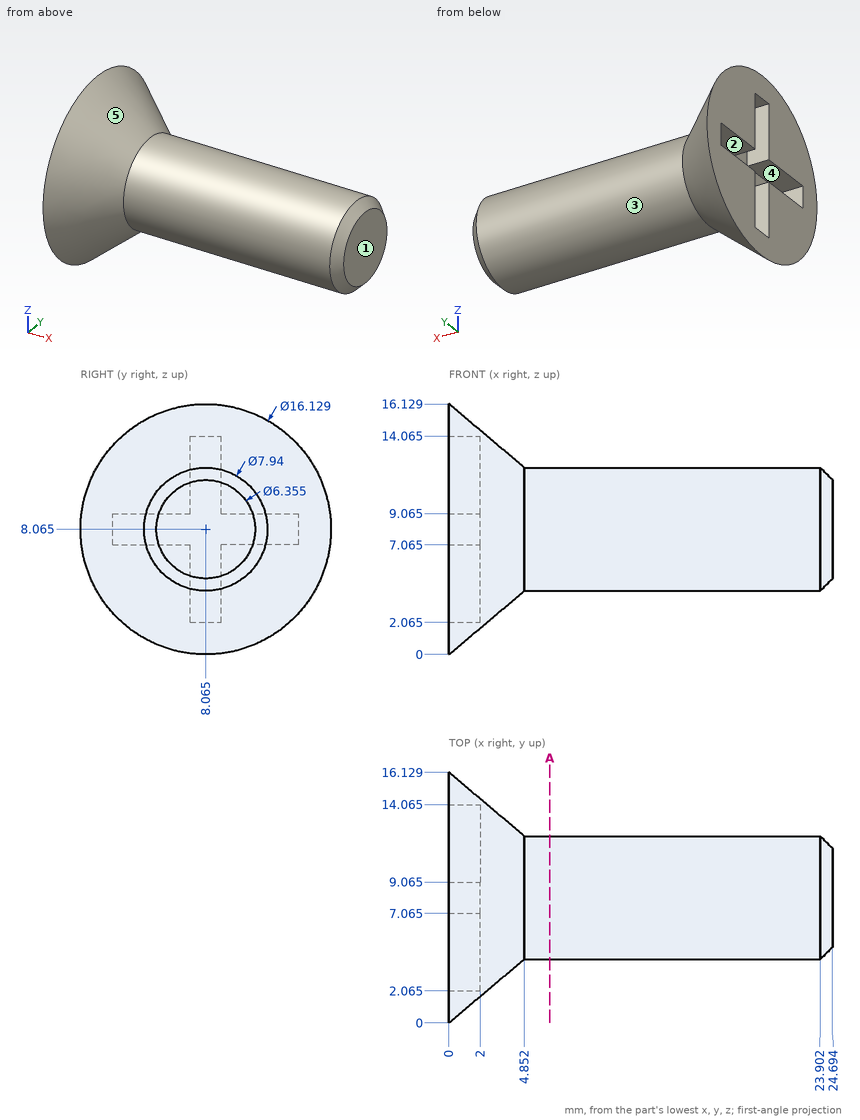
Job drawing, mm, ordinate dimensions from the low corner. One solid piece. A direction names the side the tool comes from. Coordinates: 2 decimals unless noted, no trailing zeros. Loops run counter-clockwise (first coordinate to the right, second up) from the corner with the lowest first, then second, coordinate; pieces in that order, holes last. Notation, with made-up numbers: (-35.75, 39) -> (23.25, 39) arc R9 ccw to (23.25, 50) -> close; hole circle Ø3 at (73.5, 26.5). An arc over 180 degrees is marked (long way). One line per item, written item: value.
1. Which spindle directions (+Z, -Z, +X, -X, +Y, -Y) get a long thin tool onto all of the face, cutting with end or side? Do the marked faces 4 and 5. Say none if no direction does.
Answers:
face 4: -X
face 5: +X
2. Slice it at A-A on x = 6.5. Write the cut outline in (y, z) (1 decimal), and give its area (3 significant figures).
Answers:
outline: circle Ø7.9 at (8.1, 8.1)
area: 49.5 mm^2
3. Flat gauge pins, fed straight in: P1, Ø5, axis at x = 3.5, y = 8.5, coming from the -Z side; P2, Ø0.6, axis at x = 1, y = 5, coming from the +Z side; P3, Ø1.6, axis at x = 1, z = 12, coming from the -Y side (1 decimal); P4, Ø4, axis at x = 18, z = 14.5, coming from the +Y side. Where does each tip first touch, or does it go through?
Answers:
P1: stops at z = 0.85
P2: stops at z = 14.91
P3: stops at y = 1.1
P4: passes through
4. Pull direction Y, two halves, no side cores. Call the marked faces 1, 2 and 3: pulls with the +Y half, pulls with the -Y half, needs draft (parallel to the pull), parting line crosses it, or undercut.
Answers:
face 1: needs draft
face 2: undercut
face 3: parting line crosses it
5. Drill centre lines: line 1 (Z direction, x = 1.5, y = 11.25) (1 decimal); line 2 (Z direction, x = 10.5, y = 6.25) (1 decimal); line 3 (Z direction, x = 3, y = 8.25) (1 decimal). Where is each one in solid material? Low to high. Write a range as [from, to].
Answers:
line 1: z = [2.1, 7.1], [9.1, 14.1]
line 2: z = [4.5, 11.6]
line 3: z = [2.5, 13.6]
